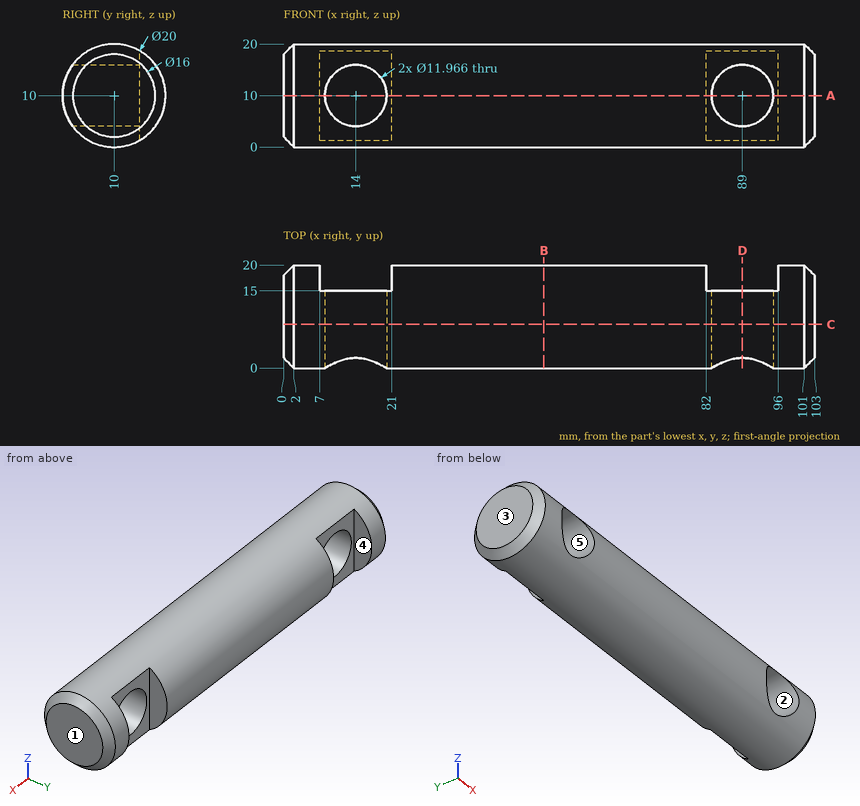
Input: dimensioned drawing with shaded views. Units: mm. Origin: part minimum x, y, z. A direction names the side the tool comes from. Round coordinates to 2 decimals unless told otherwise and drop trailing zeros. Order: outer loops, then holes, each group sorted by start corner. A loop starts at its lowest first (then second) coordinate and runs counter-clockwise, first axis right, second up. Notation, with made-up numbers: M -5,-14.75 L 1,-14.75 A10 ccw 1,1.25 Z; hole C 47.5,-34.75 d7. An arc over 180 degrees is marked long. Use one line per item in the form item = value. Start each with the question number.
Q1. Pin query (flat end, axial travel): pin 1 Ø1 at (x, z) = (45.5, 12.5) entering from +Y; pin 2 Ø11 at (x, z) = (89, 10) entering from +Y; pin 3 Ø10 at (x, z) = (50, 13) entering from +Y; pin 4 Ø3 at (x, z) = (86, 13.5) entering from -Y. Return the tip coordinate at first contact, or that it passes through.
Q2. Cut plane D-D (x = 89). Return loops of the section in (y, z), and give its area (3 significant figures).
Q3. Material intervals for line 1 (X direction, y = 5, z = 10); line 2 (X direction, y = 4.5, z = 12); line 3 (Y direction, x = 58.5, z = 2), sorted ascending. Write a range as [from, to].
Q4. Cut plane C-C (y = 8.5). Count the separate pieces of the cut face and the enclosed holes in it, and give its area (3 significant figures).
Q5. Mould query, pull axis X, two halves, no side actions, for the marked faces 1, 2 and 3. Classes: +X half, -X half, draft (parallel to the pull), parting line (faces both ways), or undercut.
Q6. Access query for the marked faces 4 and 5. Directions: +Z, -Z, +X, -X, +Y, -Y. A direction counts if a zero-diameter tool reaches every point of the face in a straight line with its end or side. Return the directions, or none.
Q7. Cut plane A-A (z = 10). Return loops of the section in (x, y).
Q8. Cut plane B-B (x = 50.5). Return loops of the section in (y, z), and give its area (3 significant figures).
Geometry results:
q1.pin_1 = 19.8
q1.pin_2 = through
q1.pin_3 = 20
q1.pin_4 = 0.86
q2.outline = M 1.99,4.02 A10 ccw 15,1.34 L 15,4.02 Z; M 1.99,15.98 L 15,15.98 L 15,18.66 A10 ccw Z
q2.area = 80.8 mm^2
q3.line_1 = [0, 8.02], [19.98, 83.02], [94.98, 103]
q3.line_2 = [0, 8.36], [19.64, 83.36], [94.64, 103]
q3.line_3 = [4, 16]
q4.separate_pieces = 1
q4.enclosed_holes = 2
q4.area = 1,800 mm^2
q5.face_1 = +X half
q5.face_2 = undercut
q5.face_3 = -X half
q6.face_4 = +Z, -Z, +Y
q6.face_5 = +Y, -Y
q7.outline = M 0,2 L 2,0 L 8.02,0 L 8.02,15 L 7,15 L 7,20 L 2,20 L 0,18 Z; M 19.98,0 L 83.02,0 L 83.02,15 L 82,15 L 82,20 L 21,20 L 21,15 L 19.98,15 Z; M 94.98,0 L 101,0 L 103,2 L 103,18 L 101,20 L 96,20 L 96,15 L 94.98,15 Z
q8.outline = C 10,10 d20
q8.area = 314 mm^2
